Design review of the part shown in the three views and the two pictorial views. Dimensions are in mm from the part's minimum x, y and z. A direction names the side the tool comes from. Round coordinates to 2 decimals unless told otherwise and drop trailing zeros. Order: outer loops, then holes, each group sorted by start corner. A loop starts at its lowest first (then second) coordinate and runs counter-clockwise, first axis right, second up.
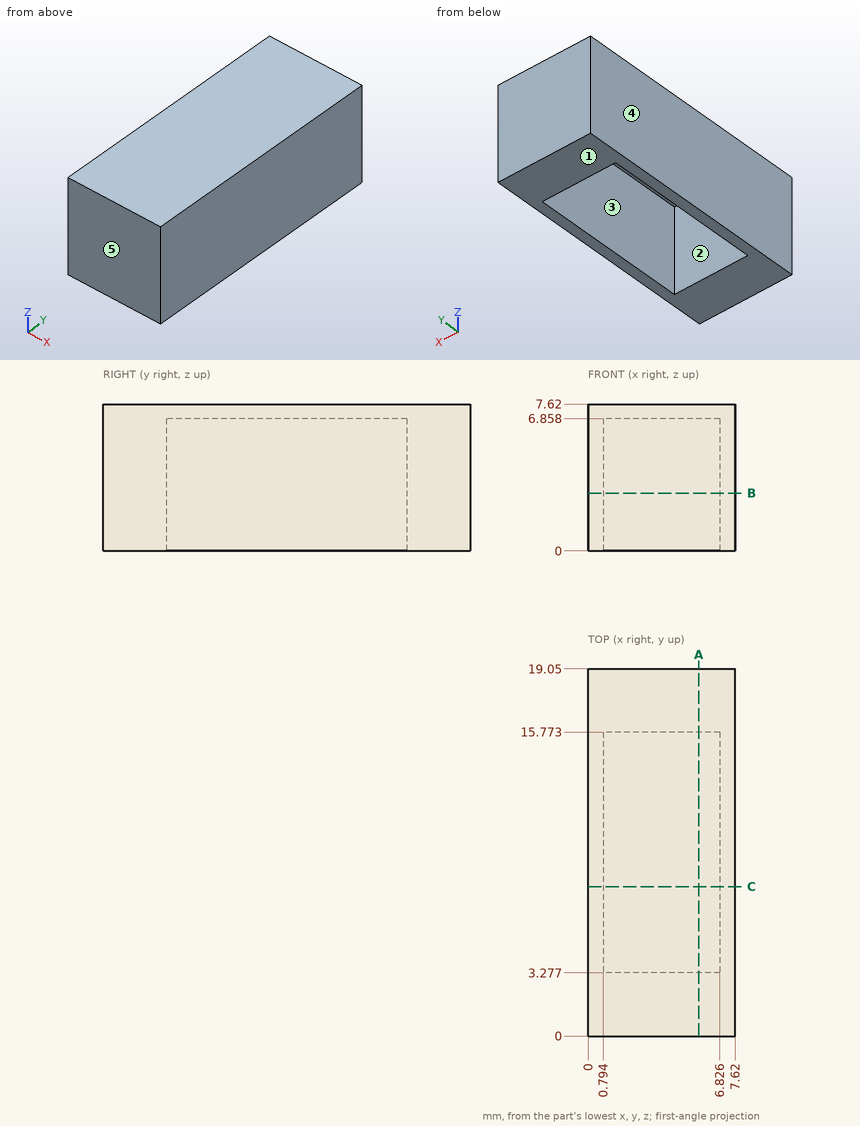
(1) Consider section A-A (x = 5.75). Write out the cut boundary in (y, z).
Data:
outline: (0, 0) - (3.28, 0) - (3.28, 6.86) - (15.77, 6.86) - (15.77, 0) - (19.05, 0) - (19.05, 7.62) - (0, 7.62) - close
(2) Insertion check: pin 1 (1.8 mm diameter, centred on x = 3.5, y = 9, fed in from -Z). The pin has a flat end and moves straight along its axis. Give the tip position at first contact, or say it passes through.
Data:
pin 1: stops at z = 6.86
(3) For the marked faces 1 and 2, list the 3-axis set-ups (+Z, -Z, +X, -X, +Y, -Y) from which the entire face can be reached by the end or side of a thin tool; tool diameter is ignored.
Data:
face 1: -Z, +X, -X, +Y, -Y
face 2: -Z
(4) Consider section C-C (y = 7.75). Write out the cut boundary in (x, z), and give its area (3 significant figures).
Data:
outline: (0, 0) - (0.79, 0) - (0.79, 6.86) - (6.83, 6.86) - (6.83, 0) - (7.62, 0) - (7.62, 7.62) - (0, 7.62) - close
area: 16.7 mm2
(5) Draft analysis for pull direction X (two halves, no side actions). For the marked faces 3, 4 and 5, state which applies: pulls with the +X half, pulls with the -X half, needs draft (parallel to the pull), parting line crosses it, or undercut.
Data:
face 3: undercut
face 4: pulls with the -X half
face 5: needs draft
(6) Consider section B-B (z = 3). Write out the cut boundary in (x, y).
Data:
outline: (0, 0) - (7.62, 0) - (7.62, 19.05) - (0, 19.05) - close; hole (0.79, 3.28) - (6.83, 3.28) - (6.83, 15.77) - (0.79, 15.77) - close
(7) To check wall thickness, follow probe 1 along Y at (x, z) = (4, 4.5); probe 2 along X at (y, z) = (15, 4.5); probe 3 along Z at (x, y) = (1.25, 3.5). State the ranges of each line that lie inside material, in increasing order.
Data:
probe 1: y = 0 to 3.28, 15.77 to 19.05
probe 2: x = 0 to 0.79, 6.83 to 7.62
probe 3: z = 6.86 to 7.62
